from build123d import *

# Parameters (mm, degrees)
SKETCH1_R           = 1.7018
SKETCH1_R_2         = 0.98425
SKETCH1_W           = 127
SKETCH1_H           = 127
BOSS_EXTRUDE1_DEPTH = 6.35


with BuildPart() as part:
    # Sketch1 → Boss-Extrude1 (new body)
    with BuildSketch(Plane(origin=(0, 0, 0), x_dir=(1, 0, 0), z_dir=(0, 1, 0))):
        Polygon((-155.3385836, 3.503957448), (-148.9885836, 3.503957448), (-148.9885836, -40.946042552), (-155.3385836, -40.946042552), (-155.3385836, -85.396042552), (-104.5385836, -85.396042552), (-104.5385836, -91.746042552), (-60.0885836, -91.746042552), (-60.0885836, -85.396042552), (-15.6385836, -85.396042552), (-15.6385836, -91.746042552), (28.8114164, -91.746042552), (28.8114164, -40.946042552), (35.1614164, -40.946042552), (35.1614164, 3.503957448), (28.8114164, 3.503957448), (28.8114164, 47.953957448), (35.1614164, 47.953957448), (35.1614164, 92.403957448), (-15.6385836, 92.403957448), (-15.6385836, 98.753957448), (-60.0885836, 98.753957448), (-60.0885836, 92.403957448), (-104.5385836, 92.403957448), (-104.5385836, 98.753957448), (-148.9885836, 98.753957448), (-148.9885836, 47.953957448), (-155.3385836, 47.953957448), align=None)
        with Locations(Location((-9.2885836, 73.353957448, 0), (0, 0, 270))):
            Circle(SKETCH1_R, mode=Mode.SUBTRACT)
        with Locations(Location((-65.889299947, -81.332042552, 0), (0, 0, 270))):
            Circle(SKETCH1_R_2, mode=Mode.SUBTRACT)
        with Locations(Location((-65.7464336, -64.124135606, 0), (0, 0, 270))):
            Circle(SKETCH1_R_2, mode=Mode.SUBTRACT)
        with Locations(Location((-54.573599947, -81.332042552, 0), (0, 0, 270))):
            Circle(SKETCH1_R_2, mode=Mode.SUBTRACT)
        with Locations(Location((-54.4307336, -64.124135606, 0), (0, 0, 270))):
            Circle(SKETCH1_R_2, mode=Mode.SUBTRACT)
        with Locations((-60.0885836, 3.503957448)):
            Rectangle(SKETCH1_W, SKETCH1_H, mode=Mode.SUBTRACT)
        with Locations(Location((-110.8885836, 73.353957448, 0), (0, 0, 270))):
            Circle(SKETCH1_R, mode=Mode.SUBTRACT)
        with Locations(Location((-95.0516836, 73.353957448, 0), (0, 0, 270))):
            Circle(SKETCH1_R, mode=Mode.SUBTRACT)
        with Locations(Location((-25.1254836, 73.353957448, 0), (0, 0, 270))):
            Circle(SKETCH1_R, mode=Mode.SUBTRACT)
    extrude(amount=BOSS_EXTRUDE1_DEPTH)


solid = part.part
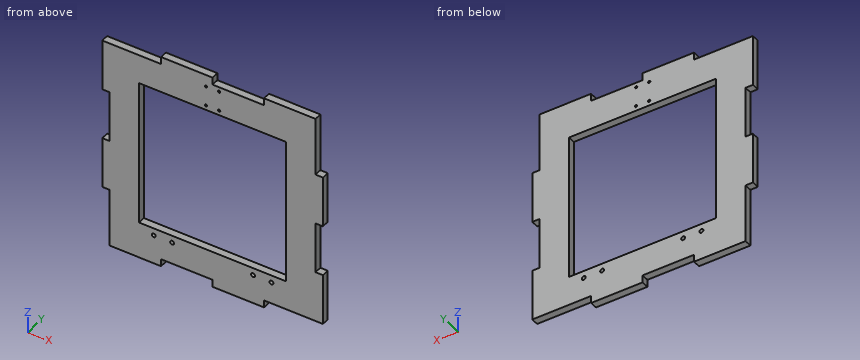
Check sheet for the modelled part. Datum: model origin and axes. Units: mm. Coordinates: 2 decimals unless noted, no trailing zeros. Write each loop counter-clockwise with the first axis right and the second up, starting at its lowest first coordinate (ties: lowest second). Pieces come first, ordered by that corner, then holes.
Item 1: Cross-section at D-D on z = -79.5. Record the boundary of the cut face in (x, y), then the cut area to 3 significant figures.
Numbers:
outline: (-148.99, 0) - (35.16, 0) - (35.16, 6.35) - (-148.99, 6.35) - close
area: 1,170 mm2
Item 2: Depth check by flat-ended pin: pin 1 Ø3 at (y, z) = (4.5, 89.5) entering from -X; pin 2 Ø1.9 at (y, z) = (4, 29.5) entering from -X; pin 3 Ø1.5 at (y, z) = (4, 68) entering from +X. Enter the tip coordinate at first touch or a pass-through.
Numbers:
pin 1: stops at x = -104.54
pin 2: stops at x = -148.99
pin 3: stops at x = 28.81
Item 3: Cross-section at A-A on x = -120.5. Record the boundary of the cut face in (y, z), then the cut area to 3 significant figures.
Numbers:
outline: (0, -98.75) - (6.35, -98.75) - (6.35, -67) - (0, -67) - close; (0, 60) - (6.35, 60) - (6.35, 85.4) - (0, 85.4) - close
area: 363 mm2
Item 4: Cross-section at C-C on y = 5.25. Count the separate pieces of the cut face and the enclosed holes in it, then the cut area to 3 significant figures.
Numbers:
separate pieces: 1
enclosed holes: 9
area: 17,700 mm2
Item 5: Cross-section at B-B on z = -17. Record the boundary of the cut face in (x, y), then the cut area to 3 significant figures.
Numbers:
outline: (-155.34, 0) - (-123.59, 0) - (-123.59, 6.35) - (-155.34, 6.35) - close; (3.41, 0) - (28.81, 0) - (28.81, 6.35) - (3.41, 6.35) - close
area: 363 mm2
Item 6: Scan lines: probe 1 along Z at (x, y) = (-25.5, 1.25); probe 2 along Z at (x, y) = (-76.5, 4.5); probe 3 along X at (y, z) = (1.5, -52). Record each from-to range of solid material in increasing order.
Numbers:
probe 1: z = -98.75 to -75.01, -71.69 to -67, 60 to 85.4
probe 2: z = -92.4 to -67, 60 to 91.75
probe 3: x = -148.99 to -123.59, 3.41 to 35.16
